Autodesk Inventor part; units mm, degrees
ref_plane "Work Plane1" through (1.525, 0, 0) normal (0, 0, 1) x (1, 0, 0)
ref_plane "YZ Plane" through (0, 0, 0) normal (1, 0, 0) x (0, 1, 0)
ref_plane "XZ Plane" through (0, 0, 0) normal (0, 1, 0) x (-1, 0, 0)
sketch "Sketch1" plane through (0, 0, 0) normal (0, 0, 1) x (1, 0, 0)
  line L0 (0, 5.5626) -> (0, 3.302)
  line L1 (25.4, 3.175) -> (44.45, 3.175)
  line L2 (44.45, 3.175) -> (44.45, 0)
  line L3 (44.45, 0) -> (-0.0001, 0)
  line L4 (-8.8901, 0) -> (53.34, 0)
  line L5 (-0.0001, 0) -> (-0.0001, 5.5626)
  line L6 (-0.0001, 5.5626) -> (0, 5.5626)
  line L7 (25.4, 3.175) -> (22.2249, 3.302)
  line L8 (22.2249, 3.302) -> (0, 3.302)
  line L9 (0, -1.1125) -> (0, 6.6751)
  dimension "d0" = 44.45
  dimension "d1" = 19.05
  dimension "d2" = 6.35
  dimension "d9" = 0.0001
  dimension "d10" = 11.1252
  dimension "d13" = 3.1751
  dimension "d14" = 6.604
revolve "Body" add sketch "Sketch1" angle 360 about axis through (44.45, 0, 0) along (-1, 0, 0)
sketch "Sketch2" plane through (-0.0001, 0, 0) normal (-1, 0, 0) x (0, 0, 1)
  line L0 (0, 6.4231) -> (5.5626, 3.2116)
  line L1 (5.5626, 3.2116) -> (5.5626, -3.2116)
  line L2 (5.5626, -3.2116) -> (0, -6.4231)
  line L3 (0, -6.4231) -> (-5.5626, -3.2116)
  line L4 (-5.5626, -3.2116) -> (-5.5626, 3.2116)
  line L5 (-5.5626, 3.2116) -> (0, 6.4231)
  point P0 (0, 0)
  point P1 (0, 0)
  dimension "d11" = 11.1252
extrude "Head" add sketch "Sketch2" along normal blind 4.7752
sketch "Sketch4" plane through (0, 0, 0) normal (0, 0, 1) x (1, 0, 0)
  line L0 (-4.7753, 5.5626) -> (-4.7753, 6.4231)
  line L1 (-4.7753, 6.4231) -> (-4.2785, 6.4231)
  line L2 (-4.2785, 6.4231) -> (-4.7753, 5.5626)
  line L3 (-5.7303, 0) -> (0.9549, 0)
  line L4 (-0.0001, 6.4231) -> (-4.7753, 6.4231)
  line L5 (-4.7753, 3.2116) -> (-4.7753, 6.4231)
  dimension "d5" = 30
  dimension "d19" = 11.1252
revolve "Chamfer1" cut sketch "Sketch4" angle 360 about axis through (-10, 0, 0) along (1, 0, 0)
thread "Thread"
chamfer "Chamfer2" distance 0.7791 distance2 0.7557 1 edges at (44.45, -3.175, 0) measured on face at (44.45, -0.7017, 0.0433)
ref_plane "Work Plane1" through (1.525, 0, 0) normal (0, 0, 1) x (1, 0, 0)
fillet "Fillet2" radius 0.762 1 edges at (0, -3.302, 0)
equation "\"d0\" = NLG"
equation "\"d1\" = GEL"
equation "\"d2\" = GD"
equation "\"d10\" = SD2"
equation "\"d14\" = BDM"
equation "\"d11\" = SW"
equation "\"d3\" = KOH - SD"
equation "\"d5\" = ANG1"
equation "\"d19\" = SW0"
equation "\"d63\" = R"
equation "\"d15\" = GEL"
equation "\"d6\" = -0.5 * SPD + 0.5 * GD"
equation "\"NLG\" = 44.45"
equation "\"GD\" = NND"
equation "\"BDM\" = 6.604"
equation "\"KOH\" = 4.7752"
equation "\"GEL\" = 19.05"
equation "\"SW\" = 11.1252"
equation "\"SW0\" = SW"
equation "\"SPD\" = GD1"
equation "\"SD2\" = SW"
equation "\"SD\" = 0"
equation "\"ANG1\" = 30deg"
equation "\"GAL\" = 3.175"
equation "\"GUL\" = 0.238 * GAL"
equation "\"R\" = 0.762"
equation "\"d62\" = -NLG - SD + GUL"
equation "\"GD1\" = 4.79184"
equation "\"THREADDIA\" = 6.35"
equation "\"TOA\" = 30deg"
equation "\"NND\" = 6.35"
equation "\"E0\" = 1.155 * SW"
properties part number "ANSI/ASME B18.2.1 - 1/4-20 UNC - 1.75" material "Steel, Mild"
Work out the finished part from the listing and answer in its coordinate system (mm). A direction names the side the tool comes from. Coordinates: 2 decimals unless noted, no trailing zeros. Write each loop counter-clockwise with the first axis right and the second up, starting at its lowest first coordinate (ties: lowest second). Pieces come first, ordered by that corner, then holes.
Q1. Which of the six approach directions +Z, -Z, +X, -X, +Y, -Y give full straight-line access (tool end or side, diameter ignored) to faces 1 (the face through (34.68, -0.69, -3.1)), 2 (the face through (-4.655, -5.772, 0.014))?
Q2. A cutting plane is placed at A-A, the plane x = 40. Give the vertices of the cut face in (y, z) (3 decimals), then the cut area to 3 significant figures.
Q3. Each of these flat-tipped pins is pushed along its axis until it touches: pin 1 Ø1 at (y, z) = (-2, -4) entering from +X; pin 2 Ø4 at (x, z) = (7.5, -3.5) entering from +Y; pin 3 Ø1 at (x, z) = (31.5, 0.5) entering from +Y (3 decimals). Where does it stop, or does it pass through?
Q4. A cutting plane is placed at B-B, the plane x = 10. Give the vertices of the cut face in (y, z).
Q5. Find the intervals of material crossed by line 1 (X direction, y = 0.5, z = 5.25); line 2 (Z direction, x = 28, y = 0.5); line 3 (X direction, y = -1.75, z = 2), in increasing order.
Findings below:
1. face 1: +X
1. face 2: -X, -Y
2. outline: circle Ø6.35 at (0, 0)
2. area: 31.7 mm2
3. pin 1: stops at x = 0.01
3. pin 2: stops at y = 2.94
3. pin 3: stops at y = 3.175
4. outline: circle Ø6.6 at (0, 0)
5. line 1: x = -4.78 to 0
5. line 2: z = -3.14 to 3.14
5. line 3: x = -4.78 to 44.2
